Print and shaded views of the part. All mm, measured from the part's lowest x, y and z. A direction names the side the tool comes from. Round coordinates to 2 decimals unless told otherwise and drop trailing zeros. Order: outer loops, then holes, each group sorted by start corner. A loop starts at its lowest first (then second) coordinate and runs counter-clockwise, first axis right, second up. Notation, with made-up numbers: (-6.5, 12.5) - (47.5, 12.5) arc R8 cw to (47.5, 25.5) - close; hole circle Ø3 at (46.25, 76). An arc over 180 degrees is marked (long way). Return JSON: item names as keys, results as strings. Group by question number.
Item 1: Saw through at D-D on x = 16.25. List the corners of the cut face in (y, z) (1 decimal).
Item 2: Saw through at A-A on z = 9.75. List the corners of the cut face in (x, y).
Item 3: Saw through at B-B on x = 11.5. List the corners of the cut face in (y, z).
Item 4: Saw through at C-C on y = 1.25. List the corners of the cut face in (x, z) (1 decimal).
Item 5: Tool access for the marked faces 1, 2 and 3: list every direction of +Z, -Z, +X, -X, +Y, -Y with a clear straight run to the whole face (end or side of a thin tool).
Item 6: Probe probe 1 along Z at (x, y) = (15.75, 1.5) (1 decimal); probe 2 along Y at (x, z) = (18.75, 4.25); probe 3 along Y at (x, z) = (8.75, 8.25). List the from-to ranges inside material, lowest first.
Item 7: Drop flat-ended pins along their axis: pin 1 (2 mm diameter, centred on x = 4, z = 11.5, fed in from -Y); pin 2 (4 mm diameter, centred on x = 8.5, y = 7, fed in from +Z); pin 3 (5 mm diameter, centred on y = 8, z = 9, fed in from +X). Give the stop position or say it passes through.
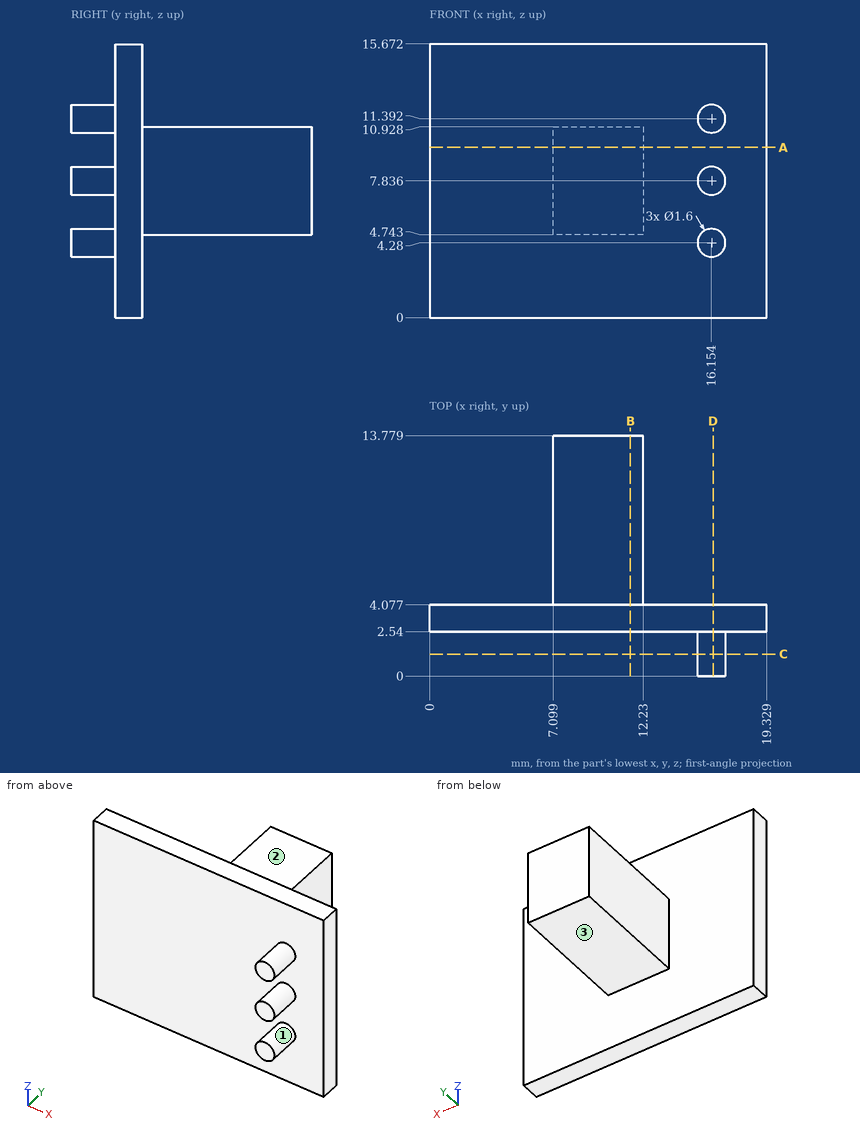
Filled in:
{
 "1": {"outline": "(0, 3.5) - (2.5, 3.5) - (2.5, 0) - (4.1, 0) - (4.1, 15.7) - (2.5, 15.7) - (2.5, 12.2) - (0, 12.2) - (0, 10.6) - (2.5, 10.6) - (2.5, 8.6) - (0, 8.6) - (0, 7) - (2.5, 7) - (2.5, 5.1) - (0, 5.1) - close"},
 "2": {"outline": "(0, 2.54) - (19.33, 2.54) - (19.33, 4.08) - (12.23, 4.08) - (12.23, 13.78) - (7.1, 13.78) - (7.1, 4.08) - (0, 4.08) - close"},
 "3": {"outline": "(2.54, 0) - (4.08, 0) - (4.08, 4.74) - (13.78, 4.74) - (13.78, 10.93) - (4.08, 10.93) - (4.08, 15.67) - (2.54, 15.67) - close"},
 "4": {"outline": "circle Ø1.6 at (16.2, 4.3); circle Ø1.6 at (16.2, 7.8); circle Ø1.6 at (16.2, 11.4)"},
 "5": {"face 1": "-Y", "face 2": "+Z, +X, -X, +Y", "face 3": "-Z, +X, -X, +Y"},
 "6": {"probe 1": "z = 3.6 to 5, 7.1 to 8.5, 10.7 to 12.1", "probe 2": "y = 2.54 to 4.08", "probe 3": "y = 2.54 to 13.78"},
 "7": {"pin 1": "stops at y = 2.54", "pin 2": "stops at z = 10.93", "pin 3": "stops at x = 12.23"}
}
